Part print with two shaded views. Sizes in mm from the minimum x, y, z corner. Round coordinates to 2 decimals unless told otherwise and drop trailing zeros. Order: outer loops, then holes, each group sorted by start corner. A loop starts at its lowest first (then second) coordinate and runs counter-clockwise, first axis right, second up. Notation, with made-up numbers: M -31,87.25 L 9,87.25 A19 cw 9,105.25 Z; hole C 83,24 d7. An arc over 180 degrees is marked long. Put each result on its own line as item: value.
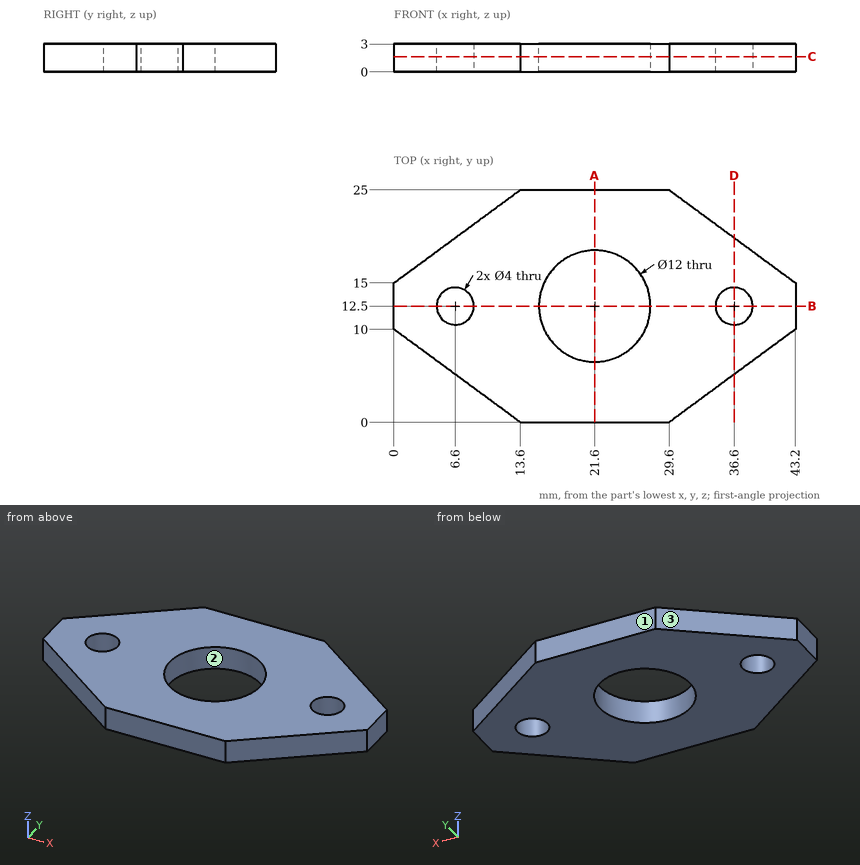
Item 1: Band-saw the part on D-D on x = 36.6. Give the cut face in (y, z), and give its area (3 significant figures).
Answers below:
outline: M 5.15,0 L 10.5,0 L 10.5,3 L 5.15,3 Z; M 14.5,0 L 19.85,0 L 19.85,3 L 14.5,3 Z
area: 32.1 mm²
Item 2: Probe line 1 along Y through (x, z) = (21.6, 2); line 2 along Y through (x, z) = (18.5, 0.6); line 3 along X through (y, z) = (8.5, 0.8). List the from-to ranges inside material, lowest first. Write a range as [from, to].
Answers below:
line 1: [0, 6.5], [18.5, 25]
line 2: [0, 7.36], [17.64, 25]
line 3: [2.04, 17.13], [26.07, 41.16]
Item 3: Pin check, flat tips, straight feed: P1, Ø1, axis at y = 17.5, z = 2, coming from the -X side; P2, Ø2.5, axis at x = 6.6, y = 12.5, coming from the +Z side. Stop position of each tip, or through.
Answers below:
P1: x = 2.72
P2: through
Item 4: Band-saw the part on C-C on z = 1.65. Give the cut face in (x, y), and give its area (3 significant figures).
Answers below:
outline: M 0,10 L 13.6,0 L 29.6,0 L 43.2,10 L 43.2,15 L 29.6,25 L 13.6,25 L 0,15 Z; hole C 6.6,12.5 d4; hole C 21.6,12.5 d12; hole C 36.6,12.5 d4
area: 670 mm²
Item 5: Band-saw the part on A-A on x = 21.6. Give the cut face in (y, z), and give its area (3 significant figures).
Answers below:
outline: M 0,0 L 6.5,0 L 6.5,3 L 0,3 Z; M 18.5,0 L 25,0 L 25,3 L 18.5,3 Z
area: 39.0 mm²
Item 6: Mould opens along X. For the marked faces 1, 2 and 3 say: pulls with the +X half, pulls with the -X half, needs draft (parallel to the pull), parting line crosses it, or undercut.
Answers below:
face 1: needs draft
face 2: undercut
face 3: pulls with the -X half
Item 7: Band-saw the part on B-B on y = 12.5. Give the cut face in (x, z), and give its area (3 significant figures).
Answers below:
outline: M 0,0 L 4.6,0 L 4.6,3 L 0,3 Z; M 8.6,0 L 15.6,0 L 15.6,3 L 8.6,3 Z; M 27.6,0 L 34.6,0 L 34.6,3 L 27.6,3 Z; M 38.6,0 L 43.2,0 L 43.2,3 L 38.6,3 Z
area: 69.6 mm²
